from build123d import *

# Parameters (mm, degrees)
SKETCH1_W           = 35
SKETCH1_H           = 45
BOSS_EXTRUDE1_DEPTH = 5
SKETCH2_R           = 1.5
CUT_EXTRUDE1_DEPTH  = 5
SKETCH4_W           = 5
SKETCH4_H           = 45
BOSS_EXTRUDE2_DEPTH = 2.5
SKETCH5_W           = 5
SKETCH5_H           = 45
BOSS_EXTRUDE3_DEPTH = 2.5
SKETCH6_R           = 1.5
CUT_EXTRUDE2_DEPTH  = 5
SKETCH7_W           = 14
SKETCH7_H           = 8
CUT_EXTRUDE3_DEPTH  = 5


with BuildPart() as part:
    # Sketch1 → Boss-Extrude1 (new body)
    with BuildSketch(Plane.XY):
        with Locations((17.5, 22.5)):
            Rectangle(SKETCH1_W, SKETCH1_H)
    extrude(amount=BOSS_EXTRUDE1_DEPTH)

    # Sketch2 → Cut-Extrude1 (cut)
    with BuildSketch(Plane.XZ):
        with Locations(Location((2, 2.5, 0), (0, 0, 270))):
            Circle(SKETCH2_R)
        with Locations(Location((33, 2.5, 0), (0, 0, 270))):
            Circle(SKETCH2_R)
        with Locations(Location((9.75, 2.5, 0), (0, 0, 270))):
            Circle(SKETCH2_R)
        with Locations(Location((25.25, 2.5, 0), (0, 0, 270))):
            Circle(SKETCH2_R)
    extrude(amount=-CUT_EXTRUDE1_DEPTH, mode=Mode.SUBTRACT)

    # Sketch4 → Boss-Extrude2 (add)
    with BuildSketch(Plane(origin=(35, 0, 0), x_dir=(0, 0, -1), z_dir=(1, 0, 0))):
        with Locations((-2.5, 22.5)):
            Rectangle(SKETCH4_W, SKETCH4_H)
    extrude(amount=BOSS_EXTRUDE2_DEPTH)

    # Sketch5 → Boss-Extrude3 (add)
    with BuildSketch(Plane.ZY):
        with Locations((2.5, 22.5)):
            Rectangle(SKETCH5_W, SKETCH5_H)
    extrude(amount=BOSS_EXTRUDE3_DEPTH)

    # Sketch6 → Cut-Extrude2 (cut)
    with BuildSketch(Plane.XY.offset(5)):
        with Locations((3.5, 36.5)):
            Circle(SKETCH6_R)
        with Locations((31.5, 8.5)):
            Circle(SKETCH6_R)
        with Locations((31.5, 36.5)):
            Circle(SKETCH6_R)
        with Locations((3.5, 8.5)):
            Circle(SKETCH6_R)
    extrude(amount=-CUT_EXTRUDE2_DEPTH, mode=Mode.SUBTRACT)

    # Sketch7 → Cut-Extrude3 (cut)
    with BuildSketch(Plane.XY.offset(5)):
        with Locations((22.5, 9.5)):
            Rectangle(SKETCH7_W, SKETCH7_H)
    extrude(amount=-CUT_EXTRUDE3_DEPTH, mode=Mode.SUBTRACT)


solid = part.part
Source: CAD feature listing. Evaluate the final solid. Frame: model axes, mm. A direction names the side the tool comes from. Coordinates: 2 decimals unless noted, no trailing zeros. Loops run counter-clockwise (first coordinate to the right, second up) from the corner with the lowest first, then second, coordinate; pieces in that order, holes last. Notation, with made-up numbers: (10, 85.25) -> (29, 85.25) arc R20 ccw to (29, 118.25) -> close; hole circle Ø11 at (-16.75, 11). An arc over 180 degrees is marked (long way). Answer in a Markdown table with one row per item. Add a question column.
Q1. Section B-B on x = 25.25. Return the cut outline in (y, z), and give its area (3 significant figures).
Q2. Ray query, line 1 along Y through (x, z) = (31.5, 1.2); line 2 along X through (y, z) = (3.9, 2.5); line 3 along Y through (x, z) = (22.5, 3.9). Return the intervals inside material, ascending.
Q3. Reachability of faces 1 (the face through (31.536, 2.465, 2.825)), 2 (the face through (37.5, 23, 3)), 3 (the face through (22, 5.5, 3)) from +Z, -Z, +X, -X, +Y, -Y: full face, straight path, thin tool, end or side. Return the list, or none.
Q4. Section D-D on z = 2.5. Return the cut outline in (x, y).
Q5. Contact query for a flat-ended pin moving along its axis: pin 1 Ø1.5 at (x, z) = (32.5, 3) entering from -Y. Output: stop coordinate, or through.
Q6. Section C-C on y = 3.5. Return the cut outline in (x, z), and give its area (3 significant figures).
Q7. Pull-direction query (Z, two-part tool) for faces 4 (the face through (18, 22, 0)), 5 (the face through (8.42, 2.46, 1.81)), 6 (the face through (18, 45, 2)); classes: pulls with the +Z half, pulls with the -Z half, needs draft (parallel to the pull), parting line crosses it, or undercut.
Q8. Section A-A on y = 8.5. Return the cut outline in (x, z).
Computed values:
| question | item | result |
|---|---|---|
| 1 | outline | (0, 0) -> (5.5, 0) -> (5.5, 5) -> (0, 5) -> (0, 4) -> (5, 4) -> (5, 1) -> (0, 1) -> close; (13.5, 0) -> (45, 0) -> (45, 5) -> (13.5, 5) -> close |
| 1 | area | 170 mm^2 |
| 2 | line 1 | y = 0 to 7, 10 to 35, 38 to 45 |
| 2 | line 2 | x = -2.5 to 0.5, 3.5 to 8.25, 11.25 to 23.75, 26.75 to 31.5, 34.5 to 37.5 |
| 2 | line 3 | y = 0 to 5.5, 13.5 to 45 |
| 3 | face 1 | -Y |
| 3 | face 2 | +Z, -Z, +X, +Y, -Y |
| 3 | face 3 | +Z, -Z |
| 4 | outline | (-2.5, 0) -> (0.5, 0) -> (0.5, 5) -> (3.5, 5) -> (3.5, 0) -> (8.25, 0) -> (8.25, 5) -> (11.25, 5) -> (11.25, 0) -> (23.75, 0) -> (23.75, 5) -> (26.75, 5) -> (26.75, 0) -> (31.5, 0) -> (31.5, 5) -> (34.5, 5) -> (34.5, 0) -> (37.5, 0) -> (37.5, 45) -> (-2.5, 45) -> close; hole circle Ø3 at (3.5, 8.5); hole circle Ø3 at (3.5, 36.5); hole (15.5, 5.5) -> (29.5, 5.5) -> (29.5, 13.5) -> (15.5, 13.5) -> close; hole circle Ø3 at (31.5, 8.5); hole circle Ø3 at (31.5, 36.5) |
| 5 | pin 1 | stops at y = 5 |
| 6 | outline | (-2.5, 0) -> (37.5, 0) -> (37.5, 5) -> (-2.5, 5) -> close; hole circle Ø3 at (2, 2.5); hole circle Ø3 at (9.75, 2.5); hole circle Ø3 at (25.25, 2.5); hole circle Ø3 at (33, 2.5) |
| 6 | area | 172 mm^2 |
| 7 | face 4 | pulls with the -Z half |
| 7 | face 5 | undercut |
| 7 | face 6 | needs draft |
| 8 | outline | (-2.5, 0) -> (2, 0) -> (2, 5) -> (-2.5, 5) -> close; (5, 0) -> (15.5, 0) -> (15.5, 5) -> (5, 5) -> close; (29.5, 0) -> (30, 0) -> (30, 5) -> (29.5, 5) -> close; (33, 0) -> (37.5, 0) -> (37.5, 5) -> (33, 5) -> close |
